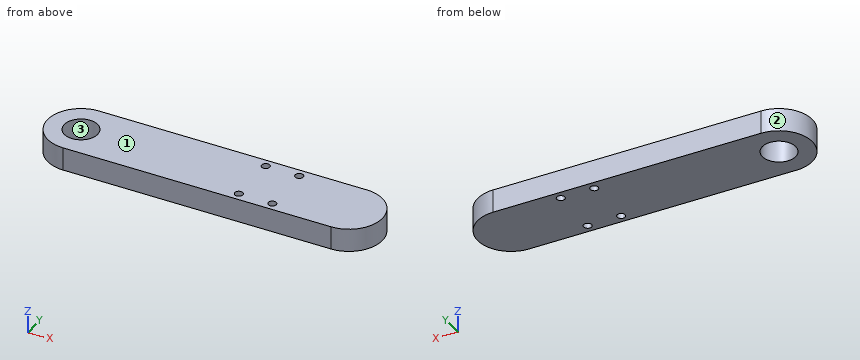
```python
from build123d import *

# Parameters (mm, degrees)
SKETCH_1_R          = 10
SKETCH_1_R_2        = 5
EXTRUDE_1_DEPTH     = 7
SKETCH_2_R          = 1.2
CUT_EXTRUDE_1_DEPTH = 10


with BuildPart() as part:
    # 草图1 → 凸台-拉伸1 (new body)
    # profile 1 of 2: a face of its own
    with BuildSketch(Plane.XY):
        Circle(SKETCH_1_R)
        Circle(SKETCH_1_R_2, mode=Mode.SUBTRACT)
    # profile 2 of 2: a face of its own
    with BuildSketch(Plane.XY):
        with BuildLine():
            Line((80, 10), (0, 10))
            ThreePointArc((0, 10), (7.071067812, 7.071067812), (10, 0))
            ThreePointArc((10, 0), (7.071067812, -7.071067812), (0, -10))
            Line((0, -10), (80, -10))
            ThreePointArc((80, -10), (90, 0), (80, 10))
        make_face()
    extrude(amount=EXTRUDE_1_DEPTH)

    # 草图2 → 切除-拉伸1 (cut)
    with BuildSketch(Plane(origin=(0, 0, 0), x_dir=(-1, 0, 0), z_dir=(0, 0, -1))):
        with Locations((-51.129038153, -7.5)):
            Circle(SKETCH_2_R)
        with Locations((-61.129038153, -7.5)):
            Circle(SKETCH_2_R)
        with Locations((-61.129038153, 7.5)):
            Circle(SKETCH_2_R)
        with Locations((-51.129038153, 7.5)):
            Circle(SKETCH_2_R)
    extrude(amount=-CUT_EXTRUDE_1_DEPTH, mode=Mode.SUBTRACT)


solid = part.part
```
CAD build for the part. Positions are in the model's coordinates, mm. Face numbers are marked on the shaded views. Give positions to 0.01 mm unless a question says otherwise; leave off trailing zeros. Loops run counter-clockwise (first coordinate to the right, second up) from the corner with the lowest first, then second, coordinate; pieces in that order, holes last. Notation, with made-up numbers: M -6,43 L 28,43 A20 ccw 28,65 Z; hole C -12.75,89.5 d5. An arc over 180 degrees is marked long. Use one line per item in the form item = value.
Item 1: Two-plate mould, pull along Y, no slides. Class the marked faces 1, 2 and 3: pulls with the +Y half, pulls with the -Y half, needs draft (parallel to the pull), parting line crosses it, or undercut.
Determined:
face_1 = needs draft
face_2 = parting line crosses it
face_3 = undercut
Item 2: Flat gauge pins, fed straight in: pin 1 (2 mm diameter, centred on x = 51.13, y = 7.5, fed in from +Z); pin 2 (1 mm diameter, centred on y = -6.5, z = 3.5, fed in from +X); pin 3 (3 mm diameter, centred on y = -2, z = 4, fed in from +X); pin 4 (1.5 mm diameter, centred on y = 2, z = 5, fed in from -X). Where does each tip first touch, or does it go through?
Determined:
pin_1 = through
pin_2 = 88
pin_3 = 89.99
pin_4 = -9.92
Item 3: Slice it at D-D (y = 7.5). List the corners of the cut face in (x, z).
Determined:
outline = M -6.61,0 L 49.93,0 L 49.93,7 L -6.61,7 Z; M 52.33,0 L 59.93,0 L 59.93,7 L 52.33,7 Z; M 62.33,0 L 86.61,0 L 86.61,7 L 62.33,7 Z
Item 4: Slice it at B-B (z = 2.5). List the corners of the cut face in (x, y).
Determined:
outline = M 0,-10 L 80,-10 A10 ccw 80,10 L 0,10 A10 ccw Z; hole C 0,0 d10; hole C 51.13,-7.5 d2.4; hole C 51.13,7.5 d2.4; hole C 61.13,-7.5 d2.4; hole C 61.13,7.5 d2.4
Item 5: Slice it at C-C (x = -2.5). List the corners of the cut face in (y, z), plus the area to 3 significant figures.
Determined:
outline = M -9.68,0 L -4.33,0 L -4.33,7 L -9.68,7 Z; M 4.33,0 L 9.68,0 L 9.68,7 L 4.33,7 Z
area = 74.9 mm2
Item 6: Drill centre lines: probe 1 along Y at (x, z) = (61, 6); probe 2 along Y at (x, z) = (0, 2.75); probe 3 along Y at (x, z) = (52, 6). Where is each one in solid material? Low to high. Write a range as from..to.
Determined:
probe_1 = -10..-8.69, -6.31..6.31, 8.69..10
probe_2 = -10..-5, 5..10
probe_3 = -10..-8.33, -6.67..6.67, 8.33..10
Item 7: Slice it at A-A (y = 0). List the corners of the cut face in (x, z).
Determined:
outline = M -10,0 L -5,0 L -5,7 L -10,7 Z; M 5,0 L 90,0 L 90,7 L 5,7 Z
